from build123d import *

# Parameters (mm, degrees)
SKETCH1_W               = 220
SKETCH1_H               = 250
SKETCH1_R               = 30
SKETCH1_R_2             = 20
SKETCH1_R_3             = 2.2
BOSS_EXTRUDE1_DEPTH     = 10
CUT_EXTRUDE1_DEPTH      = 212.187120819
CUT_EXTRUDE1_DEPTH_BACK = 212.187120819
SKETCH2_R               = 2.5
FILLET1_R               = 5
SKETCH4_R               = 1.7
CUT_EXTRUDE2_DEPTH      = 212.187120819
CIRPATTERN1_COUNT       = 4


with BuildPart() as part:
    # Sketch1 → Boss-Extrude1 (new body)
    with BuildSketch(Plane(origin=(0, 0, 0), x_dir=(1, 0, 0), z_dir=(0, 1, 0))):
        with Locations((0, -55)):
            Rectangle(SKETCH1_W, SKETCH1_H)
        with Locations(Location((0, 0, 0), (0, 0, 270))):
            Circle(SKETCH1_R, mode=Mode.SUBTRACT)
        with Locations(Location((0, -130, 0), (0, 0, 270))):
            Circle(SKETCH1_R_2, mode=Mode.SUBTRACT)
        with Locations(Location((-23.57, -106.43, 0), (0, 0, 270))):
            Circle(SKETCH1_R_3, mode=Mode.SUBTRACT)
        with Locations(Location((23.57, -106.43, 0), (0, 0, 270))):
            Circle(SKETCH1_R_3, mode=Mode.SUBTRACT)
        with Locations(Location((-23.57, -153.57, 0), (0, 0, 270))):
            Circle(SKETCH1_R_3, mode=Mode.SUBTRACT)
        with Locations(Location((23.57, -153.57, 0), (0, 0, 270))):
            Circle(SKETCH1_R_3, mode=Mode.SUBTRACT)
        with BuildLine():
            Line((-65, -77.5), (-15, -77.5))
            ThreePointArc((-15, -77.5), (-12.5, -80), (-15, -82.5))
            Line((-15, -82.5), (-65, -82.5))
            ThreePointArc((-65, -82.5), (-67.5, -80), (-65, -77.5))
        make_face(mode=Mode.SUBTRACT)
        with BuildLine():
            Line((65, -77.5), (15, -77.5))
            ThreePointArc((15, -77.5), (12.5, -80), (15, -82.5))
            Line((15, -82.5), (65, -82.5))
            ThreePointArc((65, -82.5), (67.5, -80), (65, -77.5))
        make_face(mode=Mode.SUBTRACT)
    extrude(amount=BOSS_EXTRUDE1_DEPTH)

    # Sketch2 → Cut-Extrude1 (cut, two sides: drawn at the far end of the back side and taken through both)
    with BuildSketch(Plane(origin=(0, 10, 0), x_dir=(1, 0, 0), z_dir=(0, 1, 0)).offset(-CUT_EXTRUDE1_DEPTH_BACK)):
        with Locations(Location((-100, 60, 0), (0, 0, 270))):
            Circle(SKETCH2_R)
        with Locations(Location((100, 60, 0), (0, 0, 270))):
            Circle(SKETCH2_R)
        with Locations(Location((-100, -170, 0), (0, 0, 270))):
            Circle(SKETCH2_R)
        with Locations(Location((100, -170, 0), (0, 0, 270))):
            Circle(SKETCH2_R)
        with Locations(Location((-100, -55, 0), (0, 0, 270))):
            Circle(SKETCH2_R)
        with Locations(Location((100, -55, 0), (0, 0, 270))):
            Circle(SKETCH2_R)
    extrude(amount=CUT_EXTRUDE1_DEPTH + CUT_EXTRUDE1_DEPTH_BACK, mode=Mode.SUBTRACT)

    # Fillet1
    fillet1_edges = [part.edges().sort_by_distance(p)[0] for p in [
        (-110, 5, -70),
        (110, 5, -70),
        (110, 5, 180),
        (-110, 5, 180),
    ]]
    fillet(fillet1_edges, radius=FILLET1_R)

    # Sketch4 → Cut-Extrude2 (cut, symmetric)
    with BuildSketch(Plane(origin=(0, 10, 0), x_dir=(1, 0, 0), z_dir=(0, 1, 0))):
        with Locations(Location((0, -45, 0), (0, 0, 270))):
            Circle(SKETCH4_R)
    cut_extrude2 = extrude(amount=CUT_EXTRUDE2_DEPTH, both=True, mode=Mode.SUBTRACT)

    # CirPattern1: Cut-Extrude2 ×4 about axis
    cirpattern1_axis = Axis((0, 0, 0), (0, 1, 0))
    for i in range(1, CIRPATTERN1_COUNT):
        add(cut_extrude2.rotate(cirpattern1_axis, i * 360 / CIRPATTERN1_COUNT), mode=Mode.SUBTRACT)


solid = part.part
Geometry: final body of the model. Coordinates: model frame, mm. A direction names the side the tool comes from. Round coordinates to 2 decimals unless told otherwise and drop trailing zeros. Order: outer loops, then holes, each group sorted by start corner. A loop starts at its lowest first (then second) coordinate and runs counter-clockwise, first axis right, second up. Notation, with made-up numbers: (-29.5, -13) -> (4.5, -13) arc R21 cw to (4.5, 24) -> close; hole circle Ø5 at (73.5, 70.5). An arc over 180 degrees is marked (long way). Put each result on its own line as item: value. Start each with the question number.
Q1. Section B-B on y = 3.5. Give the number of separate pieces and of enclosed holes in the cut face, and give its area (3 significant figures).
Q2. Section C-C on z = 22. Return the cut outline in (x, y).
Q3. Reachability of faces 4 (the flat face through (-40, 5, 77.5)), 5 (the cylindrical face through (108, 5, -69)) from +Z, -Z, +X, -X, +Y, -Y: full face, straight path, thin tool, end or side. Return the list, or none.
Q4. First-contact query: pin 1 (4 mm diameter, centred on x = 23.57, z = 153.57, fed in from +Y) (1 decimal). Flat tip, straight axial feed; report the tip coordinate or a pass-through.
Q5. Pull-direction query (Z, two-part tool) for faces 1 (the flat face through (-1, 5, 180)), 2 (the flat face through (-2, 10, 53)), 3 (the cylindrical face through (100.751, 4.93, 172.385)); classes: +Z half, -Z half, draft (parallel to the pull), parting line (faces both ways), or undercut.
Q6. Line query: probe 1 along Z at (x, y) = (-100, 9); probe 2 along Z at (x, y) = (48, 6); probe 3 along Z at (x, y) = (15, 3). Output: solid intervals per line, ascending.
Q7. Section A-A on z = 130. Return the cut outline in (x, y).
Ans:
1. separate pieces: 1
1. enclosed holes: 18
1. area: 50,100 mm2
2. outline: (-110, 0) -> (-20.4, 0) -> (-20.4, 10) -> (-110, 10) -> close; (20.4, 0) -> (110, 0) -> (110, 10) -> (20.4, 10) -> close
3. face 4: +Y, -Y
3. face 5: -Z, +X, +Y, -Y
4. pin 1: passes through
5. face 1: +Z half
5. face 2: draft
5. face 3: undercut
6. probe 1: z = -70 to -62.5, -57.5 to 52.5, 57.5 to 167.5, 172.5 to 180
6. probe 2: z = -70 to 77.5, 82.5 to 180
6. probe 3: z = -70 to -25.98, 25.98 to 77.5, 82.5 to 116.77, 143.23 to 180
7. outline: (-110, 0) -> (-20, 0) -> (-20, 10) -> (-110, 10) -> close; (20, 0) -> (110, 0) -> (110, 10) -> (20, 10) -> close
